Verification items for the finished model (mm, model axes). A direction names the side the tool comes from. Give positions to 0.01 mm unless a question says otherwise; leave off trailing zeros. Loops run counter-clockwise (first coordinate to the right, second up) from the corner with the lowest first, then second, coordinate; pieces in that order, holes last. Notation, with made-up numbers: M -13.5,64 L 18.5,64 A27 cw 18.5,86 Z; hole C 89.5,40 d8. An arc over 180 degrees is marked long. Answer in a Markdown table with one row per item.
```python
from build123d import *

# Parameters (mm, degrees)
SKETCH1_W           = 38.1
SKETCH1_H           = 15.24
BOSS_EXTRUDE1_DEPTH = 5.08
SKETCH2_R           = 1.651
CUT_EXTRUDE1_DEPTH  = 119.490202326
SKETCH3_W           = 12.7
SKETCH3_H           = 5.334
BOSS_EXTRUDE2_DEPTH = 30.988
SKETCH6_W           = 45.974
SKETCH6_H           = 5.334
BOSS_EXTRUDE3_DEPTH = 21.59
SKETCH7_R           = 1.778
CUT_EXTRUDE4_DEPTH  = 118.755224526
SKETCH8_R           = 3.937
CUT_EXTRUDE5_DEPTH  = 118.755224526


with BuildPart() as part:
    # Sketch1 → Boss-Extrude1 (new body)
    with BuildSketch(Plane(origin=(0, 0, 0), x_dir=(1, 0, 0), z_dir=(0, 1, 0))):
        with Locations((-81.911608108, 54.193229454)):
            Rectangle(SKETCH1_W, SKETCH1_H)
    extrude(amount=-BOSS_EXTRUDE1_DEPTH)

    # Sketch2 → Cut-Extrude1 (cut, through all)
    with BuildSketch(Plane(origin=(0, 0, 0), x_dir=(1, 0, 0), z_dir=(0, 1, 0))):
        with Locations(Location((-94.611608108, 51.907229454, 0), (0, 0, 270))):
            Circle(SKETCH2_R)
        with Locations(Location((-70.481608108, 51.907229454, 0), (0, 0, 270))):
            Circle(SKETCH2_R)
    extrude(amount=-CUT_EXTRUDE1_DEPTH, mode=Mode.SUBTRACT)

    # Sketch3 → Boss-Extrude2 (add)
    with BuildSketch(Plane(origin=(0, 0, 0), x_dir=(1, 0, 0), z_dir=(0, 1, 0))):
        with Locations((-81.911608108, 59.146229454)):
            Rectangle(SKETCH3_W, SKETCH3_H)
    extrude(amount=BOSS_EXTRUDE2_DEPTH)

    # Sketch6 → Boss-Extrude3 (add)
    with BuildSketch(Plane(origin=(0, 30.988, 0), x_dir=(1, 0, 0), z_dir=(0, 1, 0))):
        with Locations((-81.911608108, 59.146229454)):
            Rectangle(SKETCH6_W, SKETCH6_H)
    extrude(amount=BOSS_EXTRUDE3_DEPTH)

    # Sketch7 → Cut-Extrude4 (cut, through all)
    with BuildSketch(Plane.XY.offset(-56.479229454)):
        with Locations((-101.850608108, 33.655)):
            Circle(SKETCH7_R)
        with Locations((-61.972608108, 49.911)):
            Circle(SKETCH7_R)
    extrude(amount=-CUT_EXTRUDE4_DEPTH, mode=Mode.SUBTRACT)

    # Sketch8 → Cut-Extrude5 (cut, through all)
    with BuildSketch(Plane.XY.offset(-56.479229454)):
        with Locations((-81.911608108, 9.906)):
            Circle(SKETCH8_R)
    extrude(amount=-CUT_EXTRUDE5_DEPTH, mode=Mode.SUBTRACT)


solid = part.part
```
Item 1: Go/stop test with flat-tipped pins: pin 1 (5.5 mm diameter, centred on x = -101.85, y = 33.66, fed in from +Z); pin 2 (4 mm diameter, centred on y = -2, z = -52.5, fed in from -X); pin 3 (2.5 mm diameter, centred on y = 22, z = -58, fed in from +X). Record where each tip stops, or that it passes through.
Reported:
| item | result |
|---|---|
| pin 1 | stops at z = -56.48 |
| pin 2 | stops at x = -100.96 |
| pin 3 | stops at x = -75.56 |
Item 2: Sectioned sample at B-B (x = -79). Record the cut outline in (y, z).
Reported:
| item | result |
|---|---|
| outline | M -5.08,-61.81 L 7.26,-61.81 L 7.26,-56.48 L 0,-56.48 L 0,-46.57 L -5.08,-46.57 Z; M 12.56,-61.81 L 52.58,-61.81 L 52.58,-56.48 L 12.56,-56.48 Z |
Item 3: Scan lines: L1, parallel to Y at x = -68.5, z = -58; L2, parallel to Y at x = -99, z = -49.75; L3, parallel to X at y = -2, z = -55. Record each from-to range of solid material in increasing order. Write a range as [from, to].
Reported:
| item | result |
|---|---|
| L1 | y = [-5.08, 0], [30.99, 52.58] |
| L2 | y = [-5.08, 0] |
| L3 | x = [-100.96, -62.86] |
Item 4: Sectioned sample at D-D (z = -59.5). Record the cut outline in (x, y) (3 decimals), and give its area (3 significant figures).
Reported:
| item | result |
|---|---|
| outline | M -104.899,30.988 L -88.262,30.988 L -88.262,0 L -100.962,0 L -100.962,-5.08 L -62.862,-5.08 L -62.862,0 L -75.562,0 L -75.562,30.988 L -58.925,30.988 L -58.925,52.578 L -104.899,52.578 Z; hole C -101.851,33.655 d3.556; hole C -81.912,9.906 d7.874; hole C -61.973,49.911 d3.556 |
| area | 1,510 mm^2 |
Item 5: Sectioned sample at C-C (z = -51.75). Record the cut outline in (x, y).
Reported:
| item | result |
|---|---|
| outline | M -100.96,-5.08 L -96.26,-5.08 L -96.26,0 L -100.96,0 Z; M -92.97,-5.08 L -72.13,-5.08 L -72.13,0 L -92.97,0 Z; M -68.84,-5.08 L -62.86,-5.08 L -62.86,0 L -68.84,0 Z |
Item 6: Release check for a two-part mould opening along X. For faces 1 (the cylindrical face through (-68.845, -2.504, -52.122)), 2 (the flat face through (-82, 52.578, -59)), 3 (the flat face through (-75.562, 15, -59)) record: released by +X, released by -X, zero draft, split by the parting line, or undercut.
Reported:
| item | result |
|---|---|
| face 1 | undercut |
| face 2 | zero draft |
| face 3 | released by +X |
Item 7: Tool access check on faces 4 (the flat face through (-82, 0, -54)), 5 (the flat face through (-82, 32, -56.479)), 6 (the flat face through (-67, 30.988, -59)), 7 (the flat face through (-88.262, 15, -59)), 8 (the flat face through (-62.862, -3, -54)). Record the directions out of +Z, -Z, +X, -X, +Y, -Y that give a thin tool (end or side, any length) a straight path to the whole face; none if there is none.
Reported:
| item | result |
|---|---|
| face 4 | +Z |
| face 5 | +Z, +X, -X, +Y |
| face 6 | +Z, -Z, +X |
| face 7 | +Z, -Z, -X |
| face 8 | +Z, -Z, +X, -Y |
Item 8: Sectioned sample at A-A (y = 12). Record the cut outline in (x, z), and give its area (3 significant figures).
Reported:
| item | result |
|---|---|
| outline | M -88.26,-61.81 L -85.25,-61.81 L -85.25,-56.48 L -88.26,-56.48 Z; M -78.58,-61.81 L -75.56,-61.81 L -75.56,-56.48 L -78.58,-56.48 Z |
| area | 32.2 mm^2 |
